The listing builds one solid part. Answer for the finished solid, in the listing's coordinates (mm). Face numbers are marked on the shaded views. A direction names the side the tool comes from. Coordinates: 2 decimals unless noted, no trailing zeros. Order: outer loops, then holes, each group sorted by start corner. A loop starts at its lowest first (then second) coordinate and runs counter-clockwise, first axis right, second up. Notation, with made-up numbers: (2.25, -1) -> (54.25, -1) arc R26 ccw to (54.25, 21) -> close; hole circle Ø3 at (-16.75, 85). An arc over 180 degrees is marked (long way). One line per question, with ' | ' between items.
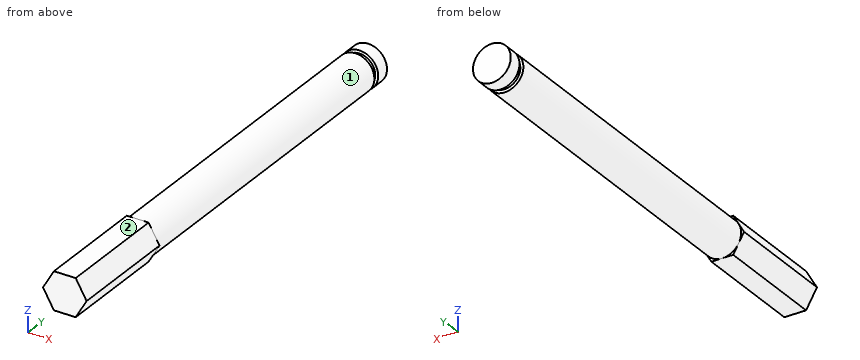
from build123d import *

# Parameters (mm, degrees)
BOSS_EXTRUDE1_DEPTH = 19.05
SKETCH2_R           = 3.175
BOSS_EXTRUDE2_DEPTH = 56.896
SKETCH3_R           = 2.667
BOSS_EXTRUDE3_DEPTH = 1.016
SKETCH4_R           = 3.175
BOSS_EXTRUDE4_DEPTH = 2.286


with BuildPart() as part:
    # Sketch1 → Boss-Extrude1 (new body)
    with BuildSketch(Plane(origin=(0, 0, 0), x_dir=(1, 0, 0), z_dir=(0, 1, 0))):
        Polygon((1.833087105, 3.175), (-1.833087105, 3.175), (-3.666174209, 0), (-1.833087105, -3.175), (1.833087105, -3.175), (3.666174209, 0), align=None)
    extrude(amount=BOSS_EXTRUDE1_DEPTH)

    # Sketch2 → Boss-Extrude2 (add)
    with BuildSketch(Plane(origin=(0, 19.05, 0), x_dir=(1, 0, 0), z_dir=(0, 1, 0))):
        with Locations(Location((0, 0, 0), (0, 0, 270))):
            Circle(SKETCH2_R)
    extrude(amount=BOSS_EXTRUDE2_DEPTH)

    # Sketch3 → Boss-Extrude3 (add)
    with BuildSketch(Plane(origin=(0, 75.946, 0), x_dir=(1, 0, 0), z_dir=(0, 1, 0))):
        with Locations(Location((0, 0, 0), (0, 0, 270))):
            Circle(SKETCH3_R)
    extrude(amount=BOSS_EXTRUDE3_DEPTH)

    # Sketch4 → Boss-Extrude4 (add)
    with BuildSketch(Plane(origin=(0, 76.962, 0), x_dir=(1, 0, 0), z_dir=(0, 1, 0))):
        with Locations(Location((0, 0, 0), (0, 0, 270))):
            Circle(SKETCH4_R)
    extrude(amount=BOSS_EXTRUDE4_DEPTH)


solid = part.part
Item 1: Each of these flat-tipped pins is pushed along its axis until it touches: pin 1 Ø0.5 at (x, z) = (2, -2.5) entering from +Y; pin 2 Ø2 at (y, z) = (66, -1.5) entering from +X; pin 3 Ø1 at (y, z) = (56, -2) entering from +X; pin 4 Ø2 at (y, z) = (62.5, -1) entering from +X (3 decimals). Where does it stop, or does it pass through?
Computed values:
pin 1: stops at y = 79.25 | pin 2: stops at x = 3.14 | pin 3: stops at x = 2.8 | pin 4: stops at x = 3.175
Item 2: Section C-C, the plane y = 60 is taken. Give the vertices of the cut face in (x, z) (3 decimals).
Computed values:
outline: circle Ø6.35 at (0, 0)
Item 3: Find the intervals of material crossed by L1, parallel to Y at x = -1, z = 2.75; L2, parallel to Z at x = 0.25, y = 67; L3, parallel to Z at x = -2.25, y = 28.5, in increasing order.
Computed values:
L1: y = 0 to 75.95, 76.96 to 79.25 | L2: z = -3.17 to 3.17 | L3: z = -2.24 to 2.24
Item 4: For the marked faces 1 and 2, determine the directions among +Z, -Z, +X, -X, +Y, -Y from which every point of the face is accessible in a straight line to the end or side of a thin tool.
Computed values:
face 1: +Y | face 2: +Z, +X, -X, +Y, -Y
Item 5: Section A-A, the plane z = 0.75 is taken. Give the vertices of the cut face in (x, y), plus the area to 3 significant figures.
Computed values:
outline: (-3.23, 0) -> (3.23, 0) -> (3.23, 19.05) -> (3.09, 19.05) -> (3.09, 75.95) -> (2.56, 75.95) -> (2.56, 76.96) -> (3.09, 76.96) -> (3.09, 79.25) -> (-3.09, 79.25) -> (-3.09, 76.96) -> (-2.56, 76.96) -> (-2.56, 75.95) -> (-3.09, 75.95) -> (-3.09, 19.05) -> (-3.23, 19.05) -> close | area: 494 mm^2
Item 6: Section B-B, the plane y = 16.5 is taken. Give the vertices of the cut face in (x, z) (3 decimals).
Computed values:
outline: (-3.666, 0) -> (-1.833, -3.175) -> (1.833, -3.175) -> (3.666, 0) -> (1.833, 3.175) -> (-1.833, 3.175) -> close
